The listing builds one solid part. Answer for the finished solid, in the listing's coordinates (mm). A direction names the side the tool comes from. Give positions to 0.01 mm unless a question says otherwise; leave off trailing zeros. Write each loop counter-clockwise with the first axis right and the second up, starting at its lowest first coordinate (ties: lowest second). Pieces come first, ordered by that corner, then holes. Notation, with made-up numbers: (-21.75, 27) - (34.25, 27) arc R24 cw to (34.25, 46) - close; hole circle Ø11 at (82, 45). An arc over 180 degrees is marked (long way). One line per item, written item: value. Start each with the question number.
from build123d import *

# Parameters (mm, degrees)
SKETCH1_W           = 177.8
SKETCH1_H           = 101.6
BOSS_EXTRUDE1_DEPTH = 12.7
BOSS_EXTRUDE2_DEPTH = 101.6
SKETCH3_R           = 6.35
CUT_EXTRUDE1_DEPTH  = 101.6
SKETCH4_W           = 25.4
SKETCH4_H           = 19.05
BOSS_EXTRUDE3_DEPTH = 101.6
SKETCH5_R           = 6.35
CUT_EXTRUDE2_DEPTH  = 101.6


with BuildPart() as part:
    # Sketch1 → Boss-Extrude1 (new body)
    with BuildSketch(Plane(origin=(0, 0, 0), x_dir=(1, 0, 0), z_dir=(0, 1, 0))):
        Rectangle(SKETCH1_W, SKETCH1_H)
    extrude(amount=BOSS_EXTRUDE1_DEPTH)

    # Sketch2 → Boss-Extrude2 (add)
    with BuildSketch(Plane.XY.offset(50.8)):
        with BuildLine():
            Line((-19.05, 0), (19.05, 0))
            ThreePointArc((19.05, 0), (0, -19.05), (-19.05, 0))
        make_face()
    extrude(amount=-BOSS_EXTRUDE2_DEPTH)

    # Sketch3 → Cut-Extrude1 (cut)
    with BuildSketch(Plane.XY.offset(50.8)):
        with Locations((0, -6.35)):
            Circle(SKETCH3_R)
    extrude(amount=-CUT_EXTRUDE1_DEPTH, mode=Mode.SUBTRACT)

    # Sketch4 → Boss-Extrude3 (add)
    with BuildSketch(Plane.XY.offset(50.8)):
        with Locations((-76.2, -9.525)):
            Rectangle(SKETCH4_W, SKETCH4_H)
    boss_extrude3 = extrude(amount=-BOSS_EXTRUDE3_DEPTH)

    # Mirror1: Boss-Extrude3 across plane
    add(boss_extrude3.mirror(Plane(origin=(0, 0, 0), x_dir=(0, 0, 1), z_dir=(1, 0, 0))))

    # Sketch5 → Cut-Extrude2 (cut)
    with BuildSketch(Plane.XY.offset(50.8)):
        with Locations((-76.2, -6.35)):
            Circle(SKETCH5_R)
        with Locations((76.2, -6.35)):
            Circle(SKETCH5_R)
    extrude(amount=-CUT_EXTRUDE2_DEPTH, mode=Mode.SUBTRACT)


solid = part.part
Item 1: Find section D-D on x = 23.5. Determine the outline of the cut face in (y, z), plus the area to 3 significant figures.
Item 2: For faces 1 (the flat face through (-63.5, -10, 1)), 2 (the cylindrical face through (69.856, -6.071, 0.711)), determine the directions among +Z, -Z, +X, -X, +Y, -Y from which every point of the face is accessible in a straight line to the end or side of a thin tool.
Item 3: Straight lines are drawn through the part: line 1 along Y through (x, z) = (-76.2, -18); line 2 along X through (y, z) = (-7.5, 40.5) (1 decimal); line 3 along X through (y, z) = (-6, -28). For each, find the intervals that lie inside material, in ascending order.
Item 4: Find section B-B on x = -76.2. Determine the outline of the cut face in (y, z).
Item 5: Find section A-A on z = 29. Determine the outline of the cut face in (x, y).
Item 6: This flat-tipped pin is pushed along its axis until it touches: pin 1 Ø13.5 at (x, z) = (-40, -10.5) entering from -Y. Where does it stop, or does it pass through?
Item 7: Find section C-C on y = -2.5. Determine the outline of the cut face in (x, z).
Values:
1. outline: (0, -50.8) - (12.7, -50.8) - (12.7, 50.8) - (0, 50.8) - close
1. area: 1,290 mm^2
2. face 1: +Z, -Z, -Y
2. face 2: +Z, -Z
3. line 1: -19.05 to -12.7, 0 to 12.7
3. line 2: -88.9 to -82.4, -70 to -63.5, -17.5 to -6.2, 6.2 to 17.5, 63.5 to 70, 82.4 to 88.9
3. line 3: -88.9 to -82.54, -69.86 to -63.5, -18.08 to -6.34, 6.34 to 18.08, 63.5 to 69.86, 82.54 to 88.9
4. outline: (-19.05, -50.8) - (-12.7, -50.8) - (-12.7, 50.8) - (-19.05, 50.8) - close; (0, -50.8) - (12.7, -50.8) - (12.7, 50.8) - (0, 50.8) - close
5. outline: (-88.9, -19.05) - (-63.5, -19.05) - (-63.5, 0) - (-19.05, 0) arc R19.05 ccw to (19.05, 0) - (63.5, 0) - (63.5, -19.05) - (88.9, -19.05) - (88.9, 12.7) - (-88.9, 12.7) - close; hole circle Ø12.7 at (-76.2, -6.35); hole circle Ø12.7 at (0, -6.35); hole circle Ø12.7 at (76.2, -6.35)
6. pin 1: y = 0
7. outline: (-88.9, -50.8) - (-81.25, -50.8) - (-81.25, 50.8) - (-88.9, 50.8) - close; (-71.15, -50.8) - (-63.5, -50.8) - (-63.5, 50.8) - (-71.15, 50.8) - close; (-18.89, -50.8) - (-5.05, -50.8) - (-5.05, 50.8) - (-18.89, 50.8) - close; (5.05, -50.8) - (18.89, -50.8) - (18.89, 50.8) - (5.05, 50.8) - close; (63.5, -50.8) - (71.15, -50.8) - (71.15, 50.8) - (63.5, 50.8) - close; (81.25, -50.8) - (88.9, -50.8) - (88.9, 50.8) - (81.25, 50.8) - close
